```python
from build123d import *

# Parameters (mm, degrees)
SKETCH1_W           = 50.8
SKETCH1_H           = 66.04
BOSS_EXTRUDE1_DEPTH = 1.778
SKETCH2_W           = 41.275
SKETCH2_H           = 5.08
BOSS_EXTRUDE2_DEPTH = 8.382
SKETCH3_R           = 1.27
BOSS_EXTRUDE3_DEPTH = 10.6426


with BuildPart() as part:
    # Sketch1 → Boss-Extrude1 (new body)
    with BuildSketch(Plane.XY):
        with Locations((25.4, 33.02)):
            Rectangle(SKETCH1_W, SKETCH1_H)
    extrude(amount=BOSS_EXTRUDE1_DEPTH)

    # Sketch2 → Boss-Extrude2 (add)
    with BuildSketch(Plane.XY.offset(1.778)):
        with Locations((25.4, 62.23)):
            Rectangle(SKETCH2_W, SKETCH2_H)
    extrude(amount=BOSS_EXTRUDE2_DEPTH)

    # Sketch3 → Boss-Extrude3 (add)
    with BuildSketch(Plane.XY.offset(1.778)):
        with Locations((12.7, 6.35)):
            Circle(SKETCH3_R)
        with Locations((38.1, 6.35)):
            Circle(SKETCH3_R)
    extrude(amount=BOSS_EXTRUDE3_DEPTH)


solid = part.part
```
Verification items for the finished model (mm, model axes). A direction names the side the tool comes from. Coordinates: 2 decimals unless noted, no trailing zeros. Write each loop counter-clockwise with the first axis right and the second up, starting at its lowest first coordinate (ties: lowest second). Pieces come first, ordered by that corner, then holes. Notation, with made-up numbers: (28, -29.5) - (73, -29.5) arc R18 ccw to (73, -25.5) - close; hole circle Ø2 at (-8.75, 51). An arc over 180 degrees is marked (long way). One line per question, with ' | ' between items. Start each with the question number.
1. Section check B-B (x = 22). Enter the section's corners in (y, z), plus the area to 3 significant figures.
2. Section check D-D (x = 38.1). Enter the section's corners in (y, z).
3. Section check C-C (z = 5.5). Enter the section's corners in (x, y).
4. Access from +Z, -Z, +X, -X, +Y, -Y to the whole of each face (thin tool, end or side, straight path). Record for faces 4 (the flat face through (25, 64.77, 6)), 5 (the flat face through (4.762, 62, 6)), 6 (the flat face through (25, 33, 0)), 7 (the flat face through (46.037, 62, 6)), 8 (the cylindrical face through (13.91, 6.73, 7.02)).
5. Gauge pin test, flat ends, axial feed: P1, Ø6.5, axis at x = 29, z = 8, coming from the -Y side; P2, Ø6, axis at x = 22.5, y = 39, coming from the +Z side; P3, Ø1.5, axis at y = 61.5, z = 4, coming from the -X side. Record the tip position at first contact, or that the pin passes through.
6. Section check A-A (y = 6.35). Enter the section's corners in (x, z), plus the area to 3 significant figures.
7. Material ranges on line 1 along X through (y, z) = (6.5, 9.5); line 2 along Z through (x, y) = (46, 17); line 3 along Y through (x, z) = (23.5, 5), recorded low to high.
8. Draft check along Y on faces 1 (the flat face through (25, 66.04, 1)), 2 (the cylindrical face through (37.164, 7.208, 7.025)), 3 (the flat face through (50.8, 33, 1)). Enter one of: released by +Y, released by -Y, zero draft, split by the parting line, or undercut.
Computed values:
1) outline: (0, 0) - (66.04, 0) - (66.04, 1.78) - (64.77, 1.78) - (64.77, 10.16) - (59.69, 10.16) - (59.69, 1.78) - (0, 1.78) - close | area: 160 mm²
2) outline: (0, 0) - (66.04, 0) - (66.04, 1.78) - (64.77, 1.78) - (64.77, 10.16) - (59.69, 10.16) - (59.69, 1.78) - (7.62, 1.78) - (7.62, 12.42) - (5.08, 12.42) - (5.08, 1.78) - (0, 1.78) - close
3) outline: (4.76, 59.69) - (46.04, 59.69) - (46.04, 64.77) - (4.76, 64.77) - close; circle Ø2.54 at (12.7, 6.35); circle Ø2.54 at (38.1, 6.35)
4) face 4: +Z, +X, -X, +Y | face 5: +Z, -X, +Y, -Y | face 6: -Z, +X, -X, +Y, -Y | face 7: +Z, +X, +Y, -Y | face 8: +Z
5) P1: y = 59.69 | P2: z = 1.78 | P3: x = 4.76
6) outline: (0, 0) - (50.8, 0) - (50.8, 1.78) - (39.37, 1.78) - (39.37, 12.42) - (36.83, 12.42) - (36.83, 1.78) - (13.97, 1.78) - (13.97, 12.42) - (11.43, 12.42) - (11.43, 1.78) - (0, 1.78) - close | area: 144 mm²
7) line 1: 11.44 to 13.96, 36.84 to 39.36 | line 2: 0 to 1.78 | line 3: 59.69 to 64.77
8) face 1: released by +Y | face 2: undercut | face 3: zero draft
